from build123d import *

# Parameters (mm, degrees)
F1_DEPTH = 20
F2_R     = 2
F3_R     = 3.5
F4_R     = 5
F6_D     = 6
F6_DEPTH = 8
F6_TIP   = 1.8025818571


with BuildPart() as f1:
    # F0 (on Top) → F1 (new body)
    with BuildSketch(Plane.XY):
        Polygon((-46.5636339205, 2.6), (-46.5636339205, 0), (-26.5636339205, 0), (-26.5636339205, 9.4), (14.2363660795, 9.4), (14.2363660795, 2.6), (-5.1636339205, 2.6), (-5.1636339205, 0), (16.8363660795, 0), (16.8363660795, 12), (-29.1636339205, 12), (-29.1636339205, 2.6), align=None)
    extrude(amount=F1_DEPTH)

    # F2
    f2_edges = [f1.edges().sort_by_distance(p)[0] for p in [
        (-29.163634, 2.6, 10),
        (14.236366, 2.6, 10),
        (14.236366, 9.4, 10),
        (-26.563634, 9.4, 10),
    ]]
    fillet(f2_edges, radius=F2_R)

    # F3
    f3_edges = [f1.edges().sort_by_distance(p)[0] for p in [
        (16.836366, 12, 10),
        (-29.163634, 12, 10),
        (-26.563634, 0, 10),
        (16.836366, 0, 10),
    ]]
    fillet(f3_edges, radius=F3_R)

    # F4
    f4_edges = [f1.edges().sort_by_distance(p)[0] for p in [
        (-46.563634, 1.3, 0),
        (-46.563634, 1.3, 20),
        (-5.163634, 1.3, 20),
        (-5.163634, 1.3, 0),
    ]]
    fillet(f4_edges, radius=F4_R)

    # F6
    with Locations(Plane.XZ):
        with Locations((-37.5636339205, 10), (5.4363660795, 10)):
            Hole(F6_D / 2, depth=F6_DEPTH)
            with Locations((0, 0, -(F6_DEPTH + F6_TIP / 2))):  # 118° drill point
                Cone(0, F6_D / 2, F6_TIP, mode=Mode.SUBTRACT)


solid = f1.part
Geometry: final body of the model. Coordinates: model frame, mm. A direction names the side the tool comes from. Give positions to 0.01 mm unless a question says otherwise; leave off trailing zeros. Order: outer loops, then holes, each group sorted by start corner. A loop starts at its lowest first (then second) coordinate and runs counter-clockwise, first axis right, second up. Notation, with made-up numbers: (87.25, -8) -> (129.25, -8) arc R18 cw to (129.25, 9) -> close; hole circle Ø10 at (-20.75, 77). An arc over 180 degrees is marked (long way). Answer as a JSON object with one key per item and string values.
Q1. Section D-D (y = 11). Output: boundary loops of the cut face in (x, z), plus the area to 3 significant figures.
Entries:
{"outline": "(-28.11, 0) -> (15.79, 0) -> (15.79, 20) -> (-28.11, 20) -> close", "area": "878 mm^2"}
Q2. Section A-A (x = -2). Output: boundary loops of the cut face in (y, z).
Entries:
{"outline": "(0, 0.35) -> (2.6, 0.35) -> (2.6, 19.65) -> (0, 19.65) -> close; (9.4, 0) -> (12, 0) -> (12, 20) -> (9.4, 20) -> close"}
Q3. First-contact query: pin 1 (5 mm diameter, centred on x = 5.44, z = 10, fed in from -Y); pin 2 (2 mm diameter, centred on y = 1.5, z = 17, fed in from +X); pin 3 (7.5 mm diameter, centred on x = -40, z = 9.5, fed in from +Y). Flat tips, straight axial feed; report the tip coordinate or a pass-through.
Entries:
{"pin 1": "stops at y = 9.4", "pin 2": "stops at x = 16.69", "pin 3": "stops at y = 2.6"}
Q4. Access query for faces 4 (the cylindrical face through (13.635, 8.83, 10.14)), 5 (the flat face through (-29.164, 7, 10)), 6 (the flat face through (-26.564, 5, 10)), 7 (the cylindrical face through (-3.66, 1.282, 1.426)). Directions: +Z, -Z, +X, -X, +Y, -Y. A direction counts if a zero-diameter tool reaches every point of the face in a straight line with its end or side. Return the directions, or none.
Entries:
{"face 4": "+Z, -Z", "face 5": "+Z, -Z, -X, +Y", "face 6": "+Z, -Z, -Y", "face 7": "-Z, -Y"}
Q5. Section B-B (z = 2.5). Output: boundary loops of the cut face in (x, y).
Entries:
{"outline": "(-45.89, 0) -> (-30.06, 0) arc R3.5 ccw to (-26.56, 3.5) -> (-26.56, 7.4) arc R2 cw to (-24.56, 9.4) -> (12.24, 9.4) arc R2 cw to (14.24, 7.4) -> (14.24, 4.6) arc R2 cw to (12.24, 2.6) -> (-4.49, 2.6) -> (-4.49, 0) -> (13.34, 0) arc R3.5 ccw to (16.84, 3.5) -> (16.84, 8.5) arc R3.5 ccw to (13.34, 12) -> (-25.66, 12) arc R3.5 ccw to (-29.16, 8.5) -> (-29.16, 4.6) arc R2 cw to (-31.16, 2.6) -> (-45.89, 2.6) -> close"}
Q6. Draft query along X for faces 1 (the flat face through (-8, 10, 20)), 2 (the flat face through (-5.164, 1, 10)), 3 (the flat face through (16.836, 6, 10)). Return one class per face: released by +X, released by -X, zero draft, split by the parting line, or undercut.
Entries:
{"face 1": "zero draft", "face 2": "undercut", "face 3": "released by +X"}
Q7. Material intervals for probe 1 along X at (y, z) = (1, 8); probe 2 along Y at (x, z) = (9.5, 15.75); probe 3 along X at (y, z) = (2.5, 8), sorted ascending.
Entries:
{"probe 1": "x = -46.56 to -39.8, -35.33 to -27.61, -5.16 to 3.2, 7.67 to 15.79", "probe 2": "y = 0 to 2.6, 9.4 to 12", "probe 3": "x = -46.56 to -39.8, -35.33 to -26.71, -5.16 to 3.2, 7.67 to 16.69"}
Q8. Section C-C (x = -21.5). Output: boundary loops of the cut face in (y, z), plus the area to 3 significant figures.
Entries:
{"outline": "(9.4, 0) -> (12, 0) -> (12, 20) -> (9.4, 20) -> close", "area": "52.0 mm^2"}
